CAD build for the part. Positions are in the model's coordinates, mm. Give positions to 0.01 mm unless a question says otherwise; leave off trailing zeros. Order: outer loops, then holes, each group sorted by start corner. A loop starts at its lowest first (then second) coordinate and runs counter-clockwise, first axis right, second up.
```python
from build123d import *

# Parameters (mm, degrees)
F1_DEPTH = 3.820417
F2_R     = 1.90733
F2_R_2   = 1.882505
F2_R_3   = 1.907323
F2_R_4   = 1.915535
F2_R_5   = 1.861563
F2_R_6   = 1.960041
F2_R_7   = 2.019149
F2_R_8   = 1.956034
F3_DEPTH = 134.979174


with BuildPart() as f1:
    # F0 (on Top) → F1 (new body)
    with BuildSketch(Plane.XY):
        Polygon((8.782074, 32.225236), (-94.263762, 30.731819), (-94.263762, 11.241347), (10.280922, 11.241347), (14.402747, 18.360883), (29.391229, 18.360883), (41.00731, 11.616066), (70.23485, 10.491922), (69.860145, 32.599941), (43.244176, 32.148832), (31.639501, 25.480404), (15.901595, 26.229829), align=None)
    extrude(amount=F1_DEPTH)

    # F2 (on Top) → F3 (join)
    with BuildSketch(Plane.XY):
        with Locations((45.582108, 28.766241)):
            Circle(F2_R)
        with Locations((51.718004, 28.766241)):
            Circle(F2_R_2)
        with Locations((56.726903, 28.766241)):
            Circle(F2_R_3)
        with Locations((61.986238, 28.641015)):
            Circle(F2_R_4)
        with Locations((61.234906, 20.877231)):
            Circle(F2_R_5)
        with Locations((59.481792, 24.759125)):
            Circle(F2_R_6)
        with Locations((54.22245, 24.633903)):
            Circle(F2_R_7)
        with Locations((48.587449, 24.633903)):
            Circle(F2_R_8)
    extrude(amount=-F3_DEPTH)


solid = f1.part
```
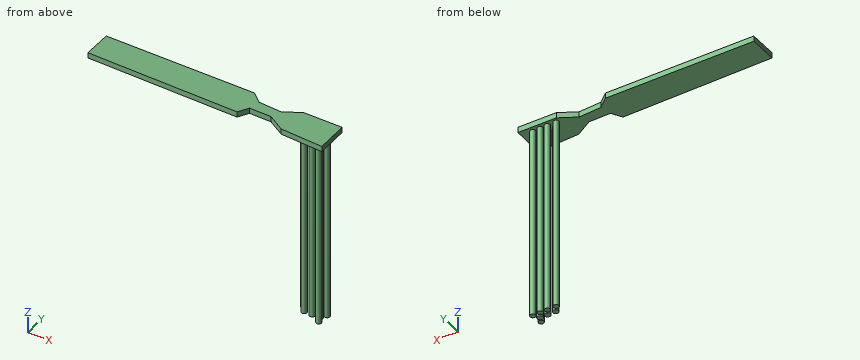
Item 1: Wall check: L1, parallel to X at y = 27.75, z = -33.5; L2, parallel to X at y = 25.5, z = -4; L3, parallel to X at y = 23, z = -111.5. Give the ranges that are in metal, low to high.
Item 2: Slice it at A-A (y = 15.75). Give the cut face in (x, z), and give its area (3 significant figures).
Item 3: Slice it at D-D (x = -19). Give the cut face in (y, z).
Item 4: Slice it at C-C (x = -47). Give the cut face in (y, z).
Item 5: Slice it at B-B (z = -102.5). Give the cut face in (x, y).
Item 6: Drop flat-ended pins along their axis: pin 1 Ø3 at (x, y) = (-45, 27) entering from -Z; pin 2 Ø3 at (x, z) = (-56.5, 2) entering from -Y; pin 3 Ø3 at (x, z) = (21.5, 1) entering from -Y. Give the stop position or say it passes through.
A:
1. L1: x = 43.97 to 47.2, 50.13 to 53.3, 55.11 to 58.34, 60.29 to 63.68
1. L2: x = 46.83 to 50.34, 52.4 to 56.05, 57.67 to 61.3
1. L3: x = 47.51 to 49.66, 53.04 to 55.41, 58.62 to 60.35
2. outline: (-94.26, 0) - (12.89, 0) - (12.89, 3.82) - (-94.26, 3.82) - close; (33.89, 0) - (70.15, 0) - (70.15, 3.82) - (33.89, 3.82) - close
2. area: 548 mm2
3. outline: (11.24, 0) - (31.82, 0) - (31.82, 3.82) - (11.24, 3.82) - close
4. outline: (11.24, 0) - (31.42, 0) - (31.42, 3.82) - (11.24, 3.82) - close
5. outline: circle Ø3.81 at (45.58, 28.77); circle Ø3.91 at (48.59, 24.63); circle Ø3.77 at (51.72, 28.77); circle Ø4.04 at (54.22, 24.63); circle Ø3.81 at (56.73, 28.77); circle Ø3.92 at (59.48, 24.76); circle Ø3.72 at (61.23, 20.88); circle Ø3.83 at (61.99, 28.64)
6. pin 1: stops at z = 0
6. pin 2: stops at y = 11.24
6. pin 3: stops at y = 18.36
